```python
from build123d import *

# Parameters (mm, degrees)
SKETCH_R     = 2.1
PAD_DEPTH    = 4.5
SKETCH001_R  = 1.9
SKETCH001_W  = 5.75
SKETCH001_H  = 15
POCKET_DEPTH = 3.2


with BuildPart() as part:
    # Sketch → Pad (new body, symmetric)
    with BuildSketch(Plane.XY):
        with BuildLine():
            Line((-5, -6), (5, -6))
            Line((5, 14.803576), (5, -6))
            ThreePointArc((8, 14.803576), (6.5, 16.303576), (5, 14.803576))
            Line((8, -14.862693), (8, 14.803576))
            ThreePointArc((7, -16.594744), (7.732051, -15.862693), (8, -14.862693))
            Line((7, -16.594744), (3.7, -18.5))
            ThreePointArc((3.7, -18.5), (4.993034, -23.462837), (9.034008, -26.620718))
            ThreePointArc((9.034008, -26.620718), (10.027512, -26.597535), (10.758643, -25.924455))
            Line((10.758643, -15.924455), (10.758643, -25.924455))
            Line((11.6, -15), (10.758643, -15.924455))
            Line((12.854013, 16.145071), (11.6, -15))
            ThreePointArc((12.854013, 16.145071), (11.054451, 20.645496), (6.5, 22.303576))
            ThreePointArc((5, 23.7), (5.446061, 22.675305), (6.5, 22.303576))
            Line((5, 25.5), (5, 23.7))
            ThreePointArc((5, 25.5), (0, 30.5), (-5, 25.5))
            Line((-5, -6), (-5, 25.5))
        make_face()
        Circle(SKETCH_R, mode=Mode.SUBTRACT)
        with BuildLine():
            ThreePointArc((-2, 23.5), (0, 21.5), (2, 23.5))
            Line((2, 23.5), (2, 26.5))
            ThreePointArc((2, 26.5), (0, 28.5), (-2, 26.5))
            Line((-2, 23.5), (-2, 26.5))
        make_face(mode=Mode.SUBTRACT)
    extrude(amount=PAD_DEPTH, both=True)

    # Sketch001 (on Face23 of Pad) → Pocket (cut)
    with BuildSketch(Plane.XY.offset(4.5)):
        with Locations((7.8, -20.5)):
            Circle(SKETCH001_R)
        with Locations((0, 12.5)):
            Rectangle(SKETCH001_W, SKETCH001_H)
    pocket = extrude(amount=-POCKET_DEPTH, mode=Mode.SUBTRACT)

    # Mirrored: Pocket across XY
    add(pocket.mirror(Plane.XY), mode=Mode.SUBTRACT)


solid = part.part
```
The model under review builds one solid part; all positions refer to its coordinate system, in mm. A direction names the side the tool comes from. Coordinates: 2 decimals unless noted, no trailing zeros. Write each loop counter-clockwise with the first axis right and the second up, starting at its lowest first coordinate (ties: lowest second). Pieces come first, ordered by that corner, then holes.
1) We need section B-B on y = 10. State the section outline as (x, z) points (3 decimals).
2) We need section D-D on y = 0. State the section outline as (x, z) points, then the cut area to 3 significant figures.
3) Machinability: for faces 1 (the face through (-2.875, 12, -3)), 2 (the face through (-2.875, 12, 3)), 3 (the face through (10.759, -21, 0)), 4 (the face through (8, 0, 0)), which of the approach directions +Z, -Z, +X, -X, +Y, -Y give a long, thin tool a straight path to every point of the face, cutting with its end or side? Answer none if there is none.
4) To check wall thickness, follow probe 1 along Y at (x, z) = (0, 2.5); probe 2 along Y at (x, z) = (7.75, 4); probe 3 along Y at (x, z) = (7, -1.5). State the ranges of each line that lie inside material, in increasing order.
5) The part is to be moulded in two halves that separate along Y. For faces 5 (the face through (11.185, -15.456, 0.063)), 6 (the face through (0, 5, 3)), 7 (the face through (-5, 10, 0)), say which applies: pulls with the +Y half, pulls with the -Y half, needs draft (parallel to the pull), parting line crosses it, or undercut.
6) Clearance check with flat-ended pins moving along their axes: pin 1 Ø3.5 at (x, y) = (7.8, -20.5) entering from -Z; pin 2 Ø2.5 at (y, z) = (-20, 0) entering from +X; pin 3 Ø1 at (y, z) = (13, -3) entering from +X. State where each tip first meets the part, or that it passes through.
7) We need section C-C on z = 3.75. State the section outline as (x, y) points (3 decimals).
8) We need section A-A on x = 0. State the section outline as (y, z) points.
Answer list:
1. outline: (-5, -4.5) - (-2.875, -4.5) - (-2.875, -1.3) - (2.875, -1.3) - (2.875, -4.5) - (5, -4.5) - (5, 4.5) - (2.875, 4.5) - (2.875, 1.3) - (-2.875, 1.3) - (-2.875, 4.5) - (-5, 4.5) - close; (8, -4.5) - (12.607, -4.5) - (12.607, 4.5) - (8, 4.5) - close
2. outline: (-5, -4.5) - (-2.1, -4.5) - (-2.1, 4.5) - (-5, 4.5) - close; (2.1, -4.5) - (5, -4.5) - (5, 4.5) - (2.1, 4.5) - close; (8, -4.5) - (12.2, -4.5) - (12.2, 4.5) - (8, 4.5) - close
2. area: 90.0 mm2
3. face 1: -Z
3. face 2: +Z
3. face 3: +Z, -Z, +X, -Y
3. face 4: +Z, -Z
4. probe 1: y = -6 to -2.1, 2.1 to 5, 20 to 21.5, 28.5 to 30.5
4. probe 2: y = -26.04 to -22.4, -18.6 to -15.83, 15.63 to 22.26
4. probe 3: y = -25.56 to -22.22, -18.78 to -16.59, 16.22 to 22.32
5. face 5: pulls with the -Y half
5. face 6: undercut
5. face 7: needs draft
6. pin 1: stops at z = -1.3
6. pin 2: stops at x = 10.76
6. pin 3: stops at x = 12.75
7. outline: (-5, -6) - (5, -6) - (5, 14.804) arc R1.5 cw to (8, 14.804) - (8, -14.863) arc R2 cw to (7, -16.595) - (3.7, -18.5) arc R8 ccw to (9.034, -26.621) arc R1.409 ccw to (10.759, -25.924) - (10.759, -15.924) - (11.6, -15) - (12.854, 16.145) arc R5.935 ccw to (6.5, 22.304) arc R1.4 cw to (5, 23.7) - (5, 25.5) arc R5 ccw to (-5, 25.5) - close; hole (-2.875, 5) - (2.875, 5) - (2.875, 20) - (-2.875, 20) - close; hole circle Ø4.2 at (0, 0); hole (-2, 23.5) arc R2 ccw to (2, 23.5) - (2, 26.5) arc R2 ccw to (-2, 26.5) - close; hole circle Ø3.8 at (7.8, -20.5)
8. outline: (-6, -4.5) - (-2.1, -4.5) - (-2.1, 4.5) - (-6, 4.5) - close; (2.1, -4.5) - (5, -4.5) - (5, -1.3) - (20, -1.3) - (20, -4.5) - (21.5, -4.5) - (21.5, 4.5) - (20, 4.5) - (20, 1.3) - (5, 1.3) - (5, 4.5) - (2.1, 4.5) - close; (28.5, -4.5) - (30.5, -4.5) - (30.5, 4.5) - (28.5, 4.5) - close
